Model file for the job. Use its own axes, mm. Face numbers are marked on the shaded views. A direction names the side the tool comes from. Round coordinates to 2 decimals unless told otherwise and drop trailing zeros. Loops run counter-clockwise (first coordinate to the right, second up) from the corner with the lowest first, then second, coordinate; pieces in that order, holes last. Notation, with made-up numbers: (51.5, 73) -> (60.5, 73) arc R15 ccw to (60.5, 97) -> close; hole circle Ø5 at (71, 68). An arc over 180 degrees is marked (long way). Use a Markdown table: item, result. Add a question column.
```python
from build123d import *

# Parameters (mm, degrees)
F1_DEPTH  = 200
F2_R      = 50
F3_DEPTH  = 50
F5_DEPTH  = 10
F7_DEPTH  = 50
F9_DEPTH  = 25
F10_W     = 200
F10_H     = 100
F11_DEPTH = 50


with BuildPart() as f1:
    # F0 (on Front) → F1 (new body)
    with BuildSketch(Plane.XZ):
        Polygon((-150, 50), (150, 50), (137.5, 0), (175, 0), (200, 100), (-200, 100), (-175, 0), (-137.5, 0), align=None)
        Polygon((175, 0), (137.5, 0), (125, -50), (-125, -50), (-137.5, 0), (-175, 0), (-150, -100), (150, -100), align=None)
    extrude(amount=-F1_DEPTH)

    # F2 (on face) → F3 (cut)
    with BuildSketch(Plane(origin=(0, 0, -100), x_dir=(1, 0, 0), z_dir=(0, 0, -1))):
        with Locations((0, -100)):
            Circle(F2_R)
    extrude(amount=-F3_DEPTH, mode=Mode.SUBTRACT)

    # F4 (on face) → F5 (join)
    with BuildSketch(Plane(origin=(0, 0, -100), x_dir=(1, 0, 0), z_dir=(0, 0, -1))):
        with BuildLine():
            ThreePointArc((50, -100), (35.3553390593, -64.6446609407), (0, -50))
            ThreePointArc((0, -50), (-35.3553390593, -135.3553390593), (50, -100))
        make_face()
        with BuildLine():
            ThreePointArc((45, -100), (-31.8198051534, -131.8198051534), (0, -55))
            ThreePointArc((0, -55), (31.8198051534, -68.1801948466), (45, -100))
        make_face(mode=Mode.SUBTRACT)
    extrude(amount=-F5_DEPTH)

    # F6 (on face) → F7 (join)
    with BuildSketch(Plane.XZ):
        Polygon((150, -100), (200, 100), (-200, 100), (-150, -100), align=None)
        Polygon((-125, -50), (-150, 50), (150, 50), (125, -50), align=None, mode=Mode.SUBTRACT)
        Polygon((150, 50), (-150, 50), (-125, -50), (125, -50), align=None)
    extrude(amount=F7_DEPTH)

    # F8 (on face) → F9 (join)
    with BuildSketch(Plane(origin=(0, 200, 0), x_dir=(-1, 0, 0), z_dir=(0, 1, 0))):
        Polygon((150, -100), (200, 100), (-200, 100), (-150, -100), align=None)
        Polygon((-125, -50), (-150, 50), (150, 50), (125, -50), align=None, mode=Mode.SUBTRACT)
        Polygon((150, 50), (-150, 50), (-125, -50), (125, -50), align=None)
    extrude(amount=F9_DEPTH)

    # F10 (on face) → F11 (cut)
    with BuildSketch(Plane.XY.offset(100)):
        with Locations((0, 50)):
            Rectangle(F10_W, F10_H)
    extrude(amount=-F11_DEPTH, mode=Mode.SUBTRACT)


solid = f1.part
```
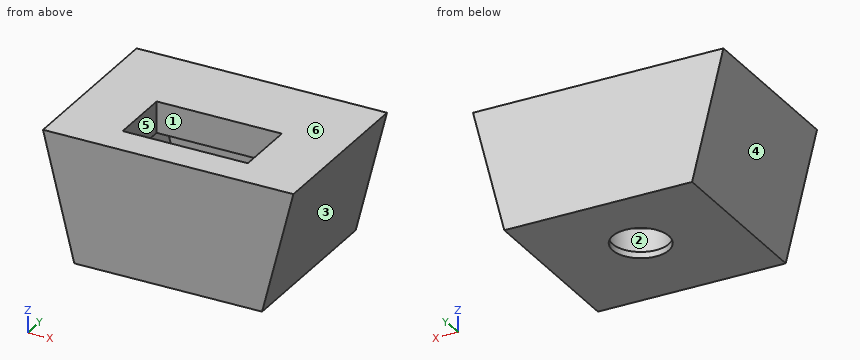
1) Tool access for the marked faces 1, 2 and 3: list every direction of +Z, -Z, +X, -X, +Y, -Y with a clear straight run to the whole face (end or side of a thin tool).
2) Pin check, flat tips, straight feed: pin 1 Ø5 at (y, z) = (34, -20) entering from +X (3 decimals); pin 2 Ø1 at (y, z) = (132.5, 47.5) entering from -X; pin 3 Ø8 at (y, z) = (118.5, -63) entering from +X. Stop position of each tip, or through.
3) Cut at B-B on x = 0. Write the cut outline in (y, z).
4) Cut at A-A on y = 188.5. Write the cut outline in (x, z), and give its area (3 significant figures).
5) Cut at C-C on z = 14. Write the cut outline in (x, y).
6) Cut at D-D on y = 43.5. Write the cut outline in (x, z), and give its area (3 significant figures).
7) Wall check: probe 1 along Y at (x, z) = (34.5, -45); probe 2 along Y at (x, z) = (-78, 71); probe 3 along Z at (x, y) = (-123, 35.5). Give the ranges that are in metal, low to high. Write a range as from..to.
8) Pull direction X, two halves, no side cores. Call the marked faces 4, 5 and 6: +X half, -X half, draft (parallel to the pull), parting line (faces both ways), or undercut.
Established:
| question | item | result |
|---|---|---|
| 1 | face 1 | +Z |
| 1 | face 2 | none |
| 1 | face 3 | -Z, +X, +Y, -Y |
| 2 | pin 1 | stops at x = 170.625 |
| 2 | pin 2 | stops at x = -187 |
| 2 | pin 3 | stops at x = 160.25 |
| 3 | outline | (-50, -100) -> (55, -100) -> (55, -90) -> (50, -90) -> (50, -50) -> (0, -50) -> (0, 100) -> (-50, 100) -> close; (100, 50) -> (200, 50) -> (200, -50) -> (150, -50) -> (150, -90) -> (145, -90) -> (145, -100) -> (225, -100) -> (225, 100) -> (100, 100) -> close |
| 4 | outline | (-200, 100) -> (-150, -100) -> (150, -100) -> (200, 100) -> close; hole (-150, 50) -> (-125, -50) -> (125, -50) -> (150, 50) -> close |
| 4 | area | 42,500 mm^2 |
| 5 | outline | (-178.5, -50) -> (178.5, -50) -> (178.5, 225) -> (-178.5, 225) -> close; hole (-141, 0) -> (141, 0) -> (141, 200) -> (-141, 200) -> close |
| 6 | outline | (-200, 100) -> (-150, -100) -> (150, -100) -> (200, 100) -> (100, 100) -> (100, 50) -> (150, 50) -> (125, -50) -> (-125, -50) -> (-150, 50) -> (-100, 50) -> (-100, 100) -> close |
| 6 | area | 32,500 mm^2 |
| 7 | probe 1 | y = -50..0, 200..225 |
| 7 | probe 2 | y = -50..0, 100..225 |
| 7 | probe 3 | z = -100..-50, 50..100 |
| 8 | face 4 | -X half |
| 8 | face 5 | undercut |
| 8 | face 6 | draft |
